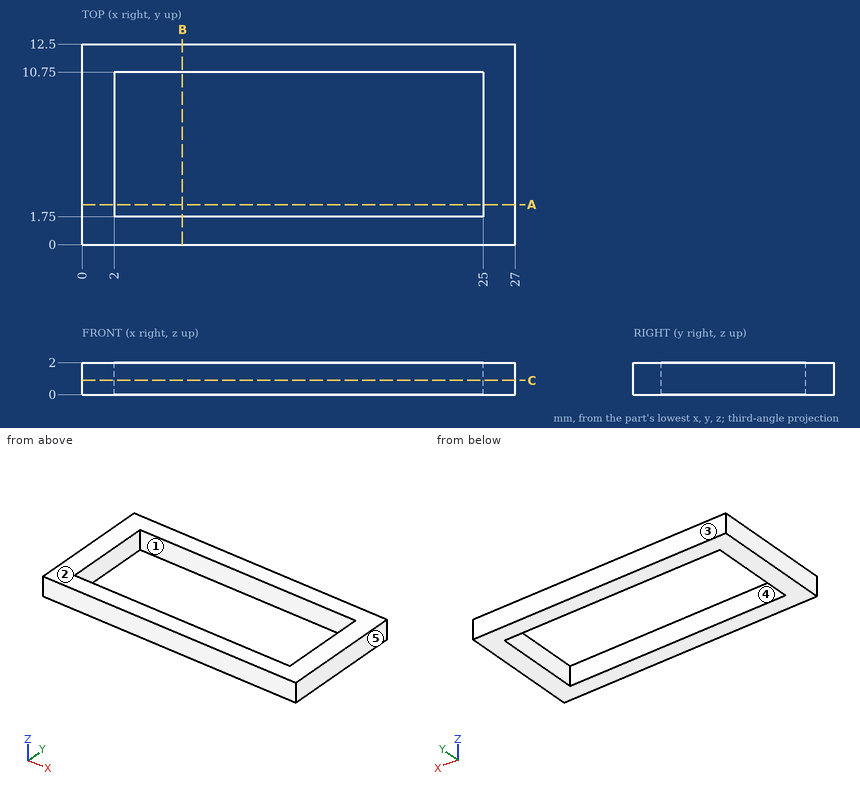
Source: three-view drawing plus pictorial views. Frame: mm from the lowest corner of the part. A direction names the side the tool comes from. Give positions to 0.01 mm unless a question says otherwise; leave off trailing zeros. Order: outer loops, then holes, each group sorted by start corner. A loop starts at its lowest first (then second) coordinate and runs counter-clockwise, first axis right, second up. Notation, with made-up numbers: (-11.75, -27.75) - (37.25, -27.75) arc R27 cw to (37.25, 5.25) - close; hole circle Ø4 at (-6.75, 43). An arc over 180 degrees is marked (long way). Answer as a JSON object with one key per item and string values. Group by question number.
Q1. Cut plane C-C, the plane z = 0.9. Output: boundary loops of the cut face in (x, y).
Q2. Cut plane B-B, the plane x = 6.25. Output: boundary loops of the cut face in (y, z).
Q3. Line query: probe 1 along Y at (x, z) = (8.5, 1.5); probe 2 along X at (y, z) = (2, 0.3). Output: solid intervals per line, ascending.
Q4. Mould query, pull axis X, two halves, no side actions, for the marked faces 3, 4 and 5. Classes: pulls with the +X half, pulls with the -X half, needs draft (parallel to the pull), parting line crosses it, or undercut.
Q5. Cut plane A-A, the plane y = 2.5. Output: boundary loops of the cut face in (x, z), then the cut area to 3 significant figures.
Q6. Set-up query: the marked faces 1 and 2. Return all of +Z, -Z, +X, -X, +Y, -Y with unobstructed straight access to the full face (end or side cutting, diameter ignored); none if empty.
Results:
{
 "1": {"outline": "(0, 0) - (27, 0) - (27, 12.5) - (0, 12.5) - close; hole (2, 1.75) - (25, 1.75) - (25, 10.75) - (2, 10.75) - close"},
 "2": {"outline": "(0, 0) - (1.75, 0) - (1.75, 2) - (0, 2) - close; (10.75, 0) - (12.5, 0) - (12.5, 2) - (10.75, 2) - close"},
 "3": {"probe 1": "0 to 1.75, 10.75 to 12.5", "probe 2": "0 to 2, 25 to 27"},
 "4": {"face 3": "needs draft", "face 4": "undercut", "face 5": "pulls with the +X half"},
 "5": {"outline": "(0, 0) - (2, 0) - (2, 2) - (0, 2) - close; (25, 0) - (27, 0) - (27, 2) - (25, 2) - close", "area": "8.00 mm^2"},
 "6": {"face 1": "+Z, -Z", "face 2": "+Z, +X, -X, +Y, -Y"}
}
